Part model, mm, in its own coordinate system. A direction names the side the tool comes from. Round coordinates to 2 decimals unless told otherwise and drop trailing zeros. Write each loop counter-clockwise with the first axis right and the second up, starting at its lowest first coordinate (ties: lowest second). Pieces come first, ordered by that corner, then holes. Notation, with made-up numbers: (29.25, -29) -> (43.25, -29) arc R19 cw to (43.25, -11) -> close; hole circle Ø3 at (66.5, -9). An arc over 180 degrees is marked (long way). Return JSON: item names as keys, results as strings. Group by question number.
```python
from build123d import *

# Parameters (mm, degrees)
F1_DEPTH = 1011.428
F3_DEPTH = 76.201
F5_DEPTH = 76.201


with BuildPart() as f1:
    # F0 (on Right) → F1 (new body)
    with BuildSketch(Plane.YZ):
        with BuildLine():
            ThreePointArc((0, 3.175), (0.9299359697, 0.9299359697), (3.175, 0))
            Line((3.175, 0), (22.225, 0))
            ThreePointArc((22.225, 0), (24.4700640303, 0.9299359697), (25.4, 3.175))
            Line((25.4, 3.175), (25.4, 73.025))
            ThreePointArc((25.4, 73.025), (24.4700640303, 75.2700640303), (22.225, 76.2))
            Line((22.225, 76.2), (3.175, 76.2))
            ThreePointArc((3.175, 76.2), (0.9299359697, 75.2700640303), (0, 73.025))
            Line((0, 73.025), (0, 3.175))
        make_face()
        with BuildLine():
            Line((19.05, 3.175), (6.35, 3.175))
            ThreePointArc((6.35, 3.175), (4.1049359697, 4.1049359697), (3.175, 6.35))
            Line((3.175, 6.35), (3.175, 69.85))
            ThreePointArc((3.175, 69.85), (4.1049359697, 72.0950640303), (6.35, 73.025))
            Line((6.35, 73.025), (19.05, 73.025))
            ThreePointArc((19.05, 73.025), (21.2950640303, 72.0950640303), (22.225, 69.85))
            Line((22.225, 69.85), (22.225, 6.35))
            ThreePointArc((22.225, 6.35), (21.2950640303, 4.1049359697), (19.05, 3.175))
        make_face(mode=Mode.SUBTRACT)
    extrude(amount=F1_DEPTH)

    # F2 (on face) → F3 (cut, through all)
    with BuildSketch(Plane(origin=(0, 0, 0), x_dir=(1, 0, 0), z_dir=(0, 0, -1))):
        Polygon((22.23230685, -3.175), (0, -3.175), (0, -22.225), (3.18230685, -22.225), align=None)
        Polygon((3.18230685, -22.225), (0, -22.225), (0, -25.40730685), align=None)
        Polygon((25.40730685, 0), (0, 0), (0, -3.175), (22.23230685, -3.175), align=None)
    extrude(amount=-F3_DEPTH, mode=Mode.SUBTRACT)

    # F4 (on face) → F5 (cut, through all)
    with BuildSketch(Plane.XY.offset(76.2)):
        Polygon((1011.428, 22.225), (1011.428, 25.4), (1008.253, 22.225), align=None)
        Polygon((1011.428, 0), (1011.428, 3.175), (989.203, 3.175), (986.028, 0), align=None)
        Polygon((1011.428, 3.175), (1011.428, 22.225), (1008.253, 22.225), (989.203, 3.175), align=None)
    extrude(amount=-F5_DEPTH, mode=Mode.SUBTRACT)


solid = f1.part
```
Item 1: Wall check: L1, parallel to Y at x = 232.5, z = 7 (3 decimals); L2, parallel to Z at x = 954.5, y = 19 (3 decimals); L3, parallel to Z at x = 277.5, y = 20. Give the ranges that are in metal, low to high.
Item 2: Which spindle directions (+Z, -Z, +X, -X, +Y, -Y) get a long thin tool onto all of the face, cutting with end or side? Do faces 1 (the face through (23, 2.41, 40.74)), 2 (the face through (499, 22.225, 39)). Say none if no direction does.
Item 3: Cut at C-C (x = 381). Write the cut outline in (y, z) (3 decimals), then the cut area to 3 significant figures.
Item 4: Two-plate mould, pull along Z, no slides. Class faces 3 (the face through (499, 13, 76.2)), 4 (the face through (499, 3.175, 38)), 5 (the face through (1009.14, 23.11, 35.46)): released by +Z, released by -Z, zero draft, split by the parting line, or undercut.
Item 5: Cut at A-A (y = 14.25). Write the cut outline in (x, z) (3 decimals), then the cut area to 3 significant figures.
Item 6: Cut at B-B (z = 45.5). Write the cut outline in (x, y) (3 decimals), then the cut area to 3 significant figures.
Item 7: Flat gauge pins, fed straight in: P1, Ø10, axis at y = 13.5, z = 36, coming from the +X side; P2, Ø1, axis at y = 22, z = 12.5, coming from the +X side. Where does each tip first touch, or does it go through?
Checks:
{
 "1": {"L1": "y = 0 to 3.175, 22.225 to 25.4", "L2": "z = 0 to 3.175, 73.025 to 76.2", "L3": "z = 0 to 3.32, 72.88 to 76.2"},
 "2": {"face 1": "+Z, -Z, -X, -Y", "face 2": "+X, -X"},
 "3": {"outline": "(0, 3.175) arc R3.175 ccw to (3.175, 0) -> (22.225, 0) arc R3.175 ccw to (25.4, 3.175) -> (25.4, 73.025) arc R3.175 ccw to (22.225, 76.2) -> (3.175, 76.2) arc R3.175 ccw to (0, 73.025) -> close; hole (3.175, 6.35) arc R3.175 ccw to (6.35, 3.175) -> (19.05, 3.175) arc R3.175 ccw to (22.225, 6.35) -> (22.225, 69.85) arc R3.175 ccw to (19.05, 73.025) -> (6.35, 73.025) arc R3.175 ccw to (3.175, 69.85) -> close", "area": "605 mm2"},
 "4": {"face 3": "released by +Z", "face 4": "undercut", "face 5": "zero draft"},
 "5": {"outline": "(11.157, 0) -> (1000.278, 0) -> (1000.278, 3.175) -> (11.157, 3.175) -> close; (11.157, 73.025) -> (1000.278, 73.025) -> (1000.278, 76.2) -> (11.157, 76.2) -> close", "area": "6,280 mm2"},
 "6": {"outline": "(0.007, 25.4) -> (3.182, 22.225) -> (1008.253, 22.225) -> (1011.428, 25.4) -> close; (22.232, 3.175) -> (25.407, 0) -> (986.028, 0) -> (989.203, 3.175) -> close", "area": "6,260 mm2"},
 "7": {"P1": "passes through", "P2": "stops at x = 1008.53"}
}
